Could you check a few things on this model? Use its own coordinates, in mm. A direction names the side the tool comes from. Round coordinates to 2 decimals unless told otherwise and drop trailing zeros. Write each loop counter-clockwise with the first axis right and the second up, starting at its lowest first coordinate (ties: lowest second). Pieces come first, ordered by that corner, then holes. Notation, with made-up numbers: M -29.5,4 L 7.5,4 A21 cw 7.5,15 Z; hole C 17.5,85 d2. An arc over 180 degrees is marked long. One line per question, with ' | ' between items. Start each with the question number.
```python
from build123d import *

# Parameters (mm, degrees)
SKETCH003_R  = 5
PAD002_DEPTH = 30
SKETCH004_R  = 2.5
PAD003_DEPTH = 15
SKETCH002_R  = 15
PAD001_DEPTH = 30
SKETCH001_R  = 2.3
SKETCH_R     = 40
PAD_DEPTH    = 5


with BuildPart() as pad002:
    # Sketch003 → Pad002 (new body)
    with BuildSketch(Plane.XY):
        Circle(SKETCH003_R)
    extrude(amount=PAD002_DEPTH)


with BuildPart() as pad003:
    # Sketch004 → Pad003 (new body, symmetric)
    with BuildSketch(Plane.XZ):
        with Locations((0, 20)):
            Circle(SKETCH004_R)
    extrude(amount=PAD003_DEPTH, both=True)


with BuildPart() as post:
    # Sketch002 → Pad001 (new body)
    with BuildSketch(Plane.XY):
        Circle(SKETCH002_R)
    extrude(amount=PAD001_DEPTH)

    # Cut002: cut Pad003
    add(pad003.part, mode=Mode.SUBTRACT)

    # Cut003: cut Pad002
    add(pad002.part, mode=Mode.SUBTRACT)


with BuildPart() as revolution:
    # Sketch001 → Revolution (revolve)
    with BuildSketch(Plane.XZ):
        with Locations((25, 5.4)):
            Circle(SKETCH001_R)
    revolve(axis=Axis((0, 0, 0), (0, 0, 1)))


with BuildPart() as fusion:
    # Sketch → Pad (new body)
    with BuildSketch(Plane.XY):
        Circle(SKETCH_R)
    extrude(amount=PAD_DEPTH)

    # Cut: cut Revolution
    add(revolution.part, mode=Mode.SUBTRACT)

    # Fusion: union post
    add(post.part)


solid = fusion.part
```
1. Suppose I cut it at A-A (x = 0). Write out the boundary of the cut face in (y, z).
2. I need wall thicknesses on line 1 along Z through (x, y) = (0, -9.5); line 2 along Y through (x, z) = (0, 10); line 3 along Z through (x, y) = (-14, 20.5). Which ranges of each line are inside material? Lowest first, please. Write a range as from..to.
3. I'm going to push flat-ended pins straight in: P1, Ø3, axis at x = -25, y = 21.5, coming from the +Z side; P2, Ø4, axis at y = -3, z = 19.5, coming from the -X side; P3, Ø12, axis at x = 23.5, z = 4, coming from the -Y side. Where does each tip first touch, or does it pass through?
4. If we mould it in two halves opening along X, with no side actions, what happens to faces 3 (the face through (0, 0, 5)), 4 (the face through (-3.252, -14.643, 17.325)), 5 (the face through (-1, 1, 0))? For each: released by +X, released by -X, zero draft, split by the parting line, or undercut.
5. Suppose I cut it at D-D (z = 11.5). Write out the boundary of the cut face in (x, y).
6. Which directions (+Z, -Z, +X, -X, +Y, -Y) give clear straight access to the entire face, cutting with the end or side of a thin tool? Please do faces 1 (the face through (-9, -26, 5)), 2 (the face through (-0.33, 9.59, 22.48)).
7. Suppose I cut it at B-B (y = 0). Write out the boundary of the cut face in (x, z).
8. Suppose I cut it at C-C (z = 20). Write out the boundary of the cut face in (x, y).
Computed:
1) outline: M -40,0 L 40,0 L 40,5 L 27.26,5 A2.3 cw 22.74,5 L 15,5 L 15,17.5 L 5,17.5 L 5,5 L -5,5 L -5,17.5 L -15,17.5 L -15,5 L -22.74,5 A2.3 cw -27.26,5 L -40,5 Z; M -15,22.5 L -5,22.5 L -5,30 L -15,30 Z; M 5,22.5 L 15,22.5 L 15,30 L 5,30 Z
2) line 1: z = 0..17.5, 22.5..30 | line 2: y = -15..-5, 5..15 | line 3: z = 0..3.11
3) P1: stops at z = 5 | P2: stops at x = -14.97 | P3: stops at y = -35.97
4) face 3: undercut | face 4: split by the parting line | face 5: zero draft
5) outline: C 0,0 d30; hole C 0,0 d10
6) face 1: +Z | face 2: +Y, -Y
7) outline: M -40,0 L 40,0 L 40,5 L 27.26,5 A2.3 cw 22.74,5 L 15,5 L 15,30 L 5,30 L 5,5 L -5,5 L -5,30 L -15,30 L -15,5 L -22.74,5 A2.3 cw -27.26,5 L -40,5 Z
8) outline: M -2.5,-14.79 L -2.5,-4.33 A5 cw -2.5,4.33 L -2.5,14.79 A15 ccw Z; M 2.5,-14.79 A15 ccw 2.5,14.79 L 2.5,4.33 A5 cw 2.5,-4.33 Z
